For this review, take the finished solid that the model builds, in its own axes (mm). A direction names the side the tool comes from. Coordinates: 2 decimals unless noted, no trailing zeros. Write each loop counter-clockwise with the first axis right and the second up, starting at its lowest first coordinate (ties: lowest second). Pieces come first, ordered by that corner, then holes.
```python
from build123d import *

# Parameters (mm, degrees)
SKETCH_1_R      = 1.5
EXTRUDE_1_DEPTH = 10
SKETCH_2_R      = 2.85
EXTRUDE_2_DEPTH = 1.65
FILLET_1_R      = 2


with BuildPart() as part:
    # 草图1 → 凸台-拉伸1 (new body)
    with BuildSketch(Plane.XY):
        Circle(SKETCH_1_R)
    extrude(amount=EXTRUDE_1_DEPTH)

    # 草图2 → 凸台-拉伸2 (add)
    with BuildSketch(Plane(origin=(0, 0, 0), x_dir=(-1, 0, 0), z_dir=(0, 0, -1))):
        Circle(SKETCH_2_R)
    extrude(amount=EXTRUDE_2_DEPTH)

    # 圆角1
    # the kernel refuses this fillet: 2 mm, written as the material it takes off along each edge
    with BuildSketch(Plane(origin=(0, 0, -1.65), x_dir=(-1, 0, 0), z_dir=(0, -1, 0))) as fillet_1_piece_1:
        with BuildLine():
            CenterArc((0.880863133, -2), FILLET_1_R, 10.078658108, 79.921341892)
            Line((0.880863133, 0), (0.880863133, 0.04))
            Line((0.880863133, 0.04), (2.85, 0.04))
            Line((2.85, 0.04), (2.89, 0))
            ThreePointArc((2.89, 0), (2.89, -0.825), (2.889382737, -1.643))
            Line((2.889382737, -1.643), (2.85, -1.65))
        make_face()
    revolve(axis=Axis((0, 0, -1.65), (0, 0, -1)), mode=Mode.SUBTRACT)


solid = part.part
```
Q1. Add section A-A (z = 6). State the section outline as (x, y) points, then the cut area to 3 significant figures.
Ans:
outline: circle Ø3 at (0, 0)
area: 7.07 mm2
Q2. For probe 1 along Z at (x, y) = (-0.9, 0.35); probe 2 along Z at (x, y) = (-0.05, -2.45); probe 3 along X at (y, z) = (-0.35, 1), list the stretches that pass through material, from the lowest coordinate up.
Ans:
probe 1: z = -1.65 to 10
probe 2: z = -0.89 to 0
probe 3: x = -1.46 to 1.46
Q3. Clearance check with a flat-ended pin moving along its axis: pin 1 Ø3 at (y, z) = (-1.5, 0.5) entering from +X. State where the tip first meets the part, or that it passes through.
Ans:
pin 1: stops at x = 2.85
Q4. Tool access review of faces 1 (the flat face through (0, 0, 10)), 2 (the cylindrical face through (-1.5, 0.07, 4.93)): name each direction out of +Z, -Z, +X, -X, +Y, -Y from which nothing blocks a thin tool from reaching the whole face with its end or side.
Ans:
face 1: +Z, +X, -X, +Y, -Y
face 2: +Z
